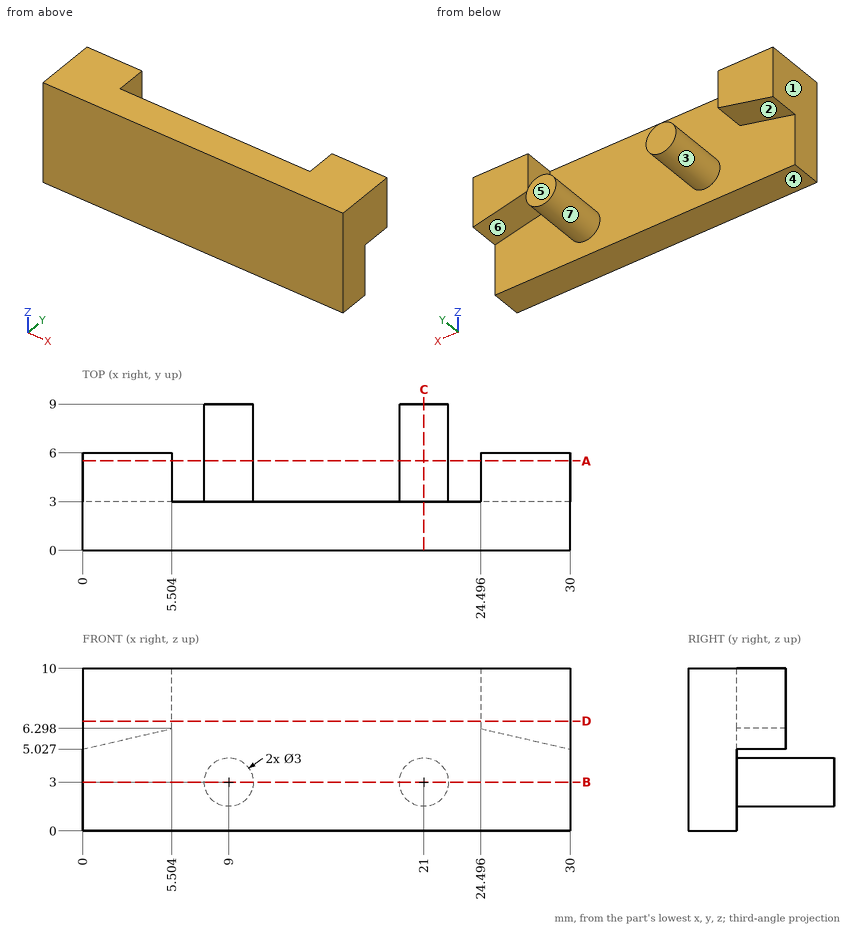
Drawing for the job (mm, zero at the part's lowest x, y, z). A direction names the side the tool comes from. Give positions to 0.01 mm unless a question says otherwise; leave off trailing zeros. Loops run counter-clockwise (first coordinate to the right, second up) from the corner with the lowest first, then second, coordinate; pieces in that order, holes last.
(1) Band-saw the part on D-D (z = 6.75). Write the cut outline in (x, y) (1 decimal), and give its area (3 significant figures).
Return value:
outline: (0, 0) - (30, 0) - (30, 6) - (24.5, 6) - (24.5, 3) - (5.5, 3) - (5.5, 6) - (0, 6) - close
area: 123 mm2
(2) Band-saw the part on C-C (x = 21). Write the cut outline in (y, z), and give its area (3 significant figures).
Return value:
outline: (0, 0) - (3, 0) - (3, 1.5) - (9, 1.5) - (9, 4.5) - (3, 4.5) - (3, 10) - (0, 10) - close
area: 48.0 mm2
(3) Pull direction X, two halves, no side cores. Call the marked faces 1, 2, 3 and 4: pulls with the +X half, pulls with the -X half, needs draft (parallel to the pull), parting line crosses it, or undercut.
Return value:
face 1: pulls with the -X half
face 2: undercut
face 3: undercut
face 4: needs draft
(4) Pin check, flat tips, straight feed: pin 1 (5.5 mm diameter, centred on x = 2.5, z = 8, fed in from +Y); pin 2 (4 mm diameter, centred on x = 16, z = 6.5, fed in from +Y); pin 3 (1.5 mm diameter, centred on x = 9, y = 6, fed in from -Z). Stop position of each tip, or through.
Return value:
pin 1: stops at y = 6
pin 2: stops at y = 3
pin 3: stops at z = 1.5
(5) Drill centre lines: line 1 along X through (y, z) = (5, 8.25) (1 decimal); line 2 along X through (y, z) = (5, 3); line 3 along Y through (x, z) = (26.25, 6). Where is each one in solid material? Low to high.
Return value:
line 1: x = 0 to 5.5, 24.5 to 30
line 2: x = 7.5 to 10.5, 19.5 to 22.5
line 3: y = 0 to 6
(6) Band-saw the part on B-B (z = 3). Write the cut outline in (x, y), and give its area (3 significant figures).
Return value:
outline: (0, 0) - (30, 0) - (30, 3) - (22.5, 3) - (22.5, 9) - (19.5, 9) - (19.5, 3) - (10.5, 3) - (10.5, 9) - (7.5, 9) - (7.5, 3) - (0, 3) - close
area: 126 mm2
(7) 3-axis set-ups, long thin cutter, end or side, ignore diameter. For the marked faces 5, 6 and 7: which of +Z, -Z, +X, -X, +Y, -Y reach the whole face in a straight line?
Return value:
face 5: +Z, -Z, +X, -X, +Y
face 6: -Z, +Y
face 7: +Y
(8) Band-saw the part on A-A (y = 5.5). Write the cut outline in (x, z) (1 decimal).
Return value:
outline: (0, 5) - (5.5, 6.3) - (5.5, 10) - (0, 10) - close; circle Ø3 at (9, 3); circle Ø3 at (21, 3); (24.5, 6.3) - (30, 5) - (30, 10) - (24.5, 10) - close
